from build123d import *

# Parameters (mm, degrees)
F0_R     = 5
F1_DEPTH = 3
F2_R     = 4
F3_DEPTH = 3
F4_R     = 3
F5_DEPTH = 3
F6_R     = 2.5
F7_DEPTH = 3
F8_R     = 2
F9_DEPTH = 3


with BuildPart() as f1:
    # F0 (on Top) → F1 (new body)
    with BuildSketch(Plane.XY):
        Circle(F0_R)
    extrude(amount=F1_DEPTH)

    # F2 (on face) → F3 (join)
    with BuildSketch(Plane.XY.offset(3)):
        Circle(F2_R)
    extrude(amount=F3_DEPTH)

    # F4 (on face) → F5 (join)
    with BuildSketch(Plane.XY.offset(6)):
        Circle(F4_R)
    extrude(amount=F5_DEPTH)

    # F6 (on face) → F7 (join)
    with BuildSketch(Plane.XY.offset(9)):
        Circle(F6_R)
    extrude(amount=F7_DEPTH)

    # F8 (on face) → F9 (join)
    with BuildSketch(Plane.XY.offset(12)):
        Circle(F8_R)
    extrude(amount=F9_DEPTH)


solid = f1.part
Design review of the part built by this model. Coordinates are the model's own, in mm. A direction names the side the tool comes from. Coordinates: 2 decimals unless noted, no trailing zeros. Order: outer loops, then holes, each group sorted by start corner. A loop starts at its lowest first (then second) coordinate and runs counter-clockwise, first axis right, second up. Notation, with made-up numbers: (11, 13.25) - (44, 13.25) arc R11 cw to (44, 18.25) - close; hole circle Ø1 at (45.25, 61.5). An arc over 180 degrees is marked (long way). Put each result on its own line as item: value.
1) Take a section at D-D, the plane x = -3.25. Give the boundary of the cut face in (y, z).
Response values:
outline: (-3.8, 0) - (3.8, 0) - (3.8, 3) - (2.33, 3) - (2.33, 6) - (-2.33, 6) - (-2.33, 3) - (-3.8, 3) - close
2) Take a section at A-A, the plane x = 0. Give the boundary of the cut face in (y, z), and give its area (3 significant figures).
Response values:
outline: (-5, 0) - (5, 0) - (5, 3) - (4, 3) - (4, 6) - (3, 6) - (3, 9) - (2.5, 9) - (2.5, 12) - (2, 12) - (2, 15) - (-2, 15) - (-2, 12) - (-2.5, 12) - (-2.5, 9) - (-3, 9) - (-3, 6) - (-4, 6) - (-4, 3) - (-5, 3) - close
area: 99.0 mm²
3) Take a section at C-C, the plane z = 7.5. Give the boundary of the cut face in (x, y).
Response values:
outline: circle Ø6 at (0, 0)
4) Tool access review of faces 1 (the face through (0, 0, 0)), 2 (the face through (-3, 0, 7)): name each direction out of +Z, -Z, +X, -X, +Y, -Y from which nothing blocks a thin tool from reaching the whole face with its end or side.
Response values:
face 1: -Z, +X, -X, +Y, -Y
face 2: +Z
5) Wall thickness on L1, parallel to Z at x = -2.25, y = -2.75; L2, parallel to Z at x = 1, y = 2; L3, parallel to X at y = -2, z = 0.75: over which ranges is each line inside the solid? List them lowest first. Write a range as from..to.
Response values:
L1: z = 0..6
L2: z = 0..12
L3: x = -4.58..4.58
6) Insertion check: P1, Ø6, axis at x = 2, y = -1.5, coming from the -Z side; P2, Ø1, axis at y = -4, z = 5.5, coming from the -X side. Each pin has a flat end and moves straight along its axis. Give the tip position at first contact, or say it passes through.
Response values:
P1: stops at z = 0
P2: stops at x = -1.94
